Autodesk Inventor part; units mm, degrees
ref_plane "YZ Plane" through (0, 0, 0) normal (1, 0, 0) x (0, 1, 0)
ref_plane "XZ Plane" through (0, 0, 0) normal (0, 1, 0) x (-1, 0, 0)
ref_plane "XY Plane" through (0, 0, 0) normal (0, 0, 1) x (1, 0, 0)
sketch "Sketch1" plane through (0, 0, 0) normal (0, 0, 1) x (1, 0, 0)
  point P0 (0, 0)
sketch "Sketch2" plane through (0, 0, 0) normal (0, 0, 1) x (1, 0, 0)
  line L0 (-52.4998, -67.5002) -> (52.4998, -67.5002)
  line L1 (52.4998, -67.5002) -> (52.4998, 67.5002)
  line L2 (52.4998, 67.5002) -> (-52.4998, 67.5002)
  line L3 (-52.4998, 67.5002) -> (-52.4998, -67.5002)
  circle A0 centre (48, 60) radius 1.5002
  circle A1 centre (-48, 60) radius 1.5002
  circle A2 centre (-48, -60) radius 1.5002
  circle A3 centre (48, -60) radius 1.5002
  circle A4 centre (22, 60) radius 1.4999
  circle A5 centre (-22, 60) radius 1.4999
  circle A6 centre (22, -60) radius 1.4999
  circle A7 centre (-22, -60) radius 1.4999
  line L4 (0, -44.9999) -> (0, 44.9999)
  line L5 (30, -44.9999) -> (30, 44.9999)
  line L6 (30, 44.9999) -> (52.4998, 54.3179)
  line L7 (30, -44.9999) -> (52.4998, -54.3208)
  line L8 (-30, -44.9999) -> (-30, 44.9999)
  line L9 (-30, 44.9999) -> (-52.4998, 54.3179)
  line L10 (-30, -44.9999) -> (-52.4998, -54.3208)
extrude "Extrusion3" add sketch "Sketch2" along normal blind 3
fillet "Fillet4" radius 4 4 edges at (-52.4998, 67.5002, 1.5) (52.4998, 67.5002, 1.5) (52.4998, -67.5002, 1.5) (-52.4998, -67.5002, 1.5)
extrude "Extrusion4" cut sketch "Sketch2" along normal blind 10 contours L3 L9 L8 L10 | L7 L5 L6 L1
fillet "Fillet5" radius 4 8 edges at (52.4998, 54.3179, 1.5) (30, 44.9999, 1.5) (-30, 44.9999, 1.5) (-52.4998, 54.3179, 1.5) (-30, -44.9999, 1.5) (-52.4998, -54.3208, 1.5) (30, -44.9999, 1.5) (52.4998, -54.3208, 1.5)
properties part number "Controller - Power Board v2"
Part model, mm, in its own coordinate system. A direction names the side the tool comes from. Coordinates: 2 decimals unless noted, no trailing zeros. Write each loop counter-clockwise with the first axis right and the second up, starting at its lowest first coordinate (ties: lowest second). Pieces come first, ordered by that corner, then holes. Notation, with made-up numbers: M -19,74 L 37,74 A24 cw 37,102 Z; hole C -12,-15.75 d11. An arc over 180 degrees is marked long. Return JSON: item names as keys, results as strings.
1. Flat gauge pins, fed straight in: pin 1 Ø2.5 at (x, y) = (-48, 60) entering from -Z; pin 2 Ø1 at (y, z) = (-18, 2.5) entering from -X. Where does each tip first touch, or does it go through?
Determined:
{"pin 1": "through", "pin 2": "x = -30"}
2. Probe L1, parallel to Y at x = 22, z = 0.95; L2, parallel to Y at x = 48, z = 1.55; L3, parallel to X at y = 59, z = 0.3. List the from-to ranges inside material, lowest first.
Determined:
{"L1": "-67.5 to -61.5, -58.5 to 58.5, 61.5 to 67.5", "L2": "-67.5 to -61.5, -58.5 to -52.46, 52.45 to 58.5, 61.5 to 67.5", "L3": "-52.5 to -49.12, -46.88 to -23.12, -20.88 to 20.88, 23.12 to 46.88, 49.12 to 52.5"}
3. 3-axis set-ups, long thin cutter, end or side, ignore diameter. For faces 1 (the face through (-51.297, 66.36, 1.521)), 2 (the face through (-30, -1, 1)), 3 (the face through (30, -1, 1)): which of +Z, -Z, +X, -X, +Y, -Y reach the whole face in a straight line?
Determined:
{"face 1": "+Z, -Z, -X, +Y", "face 2": "+Z, -Z, -X", "face 3": "+Z, -Z, +X"}
4. Saw through at B-B, the plane y = -60. Write the cut outline in (x, z).
Determined:
{"outline": "M -52.5,0 L -49.5,0 L -49.5,3 L -52.5,3 Z; M -46.5,0 L -23.5,0 L -23.5,3 L -46.5,3 Z; M -20.5,0 L 20.5,0 L 20.5,3 L -20.5,3 Z; M 23.5,0 L 46.5,0 L 46.5,3 L 23.5,3 Z; M 49.5,0 L 52.5,0 L 52.5,3 L 49.5,3 Z"}
5. Saw through at A-A, the plane x = -22. Write the cut outline in (y, z), then the cut area to 3 significant figures.
Determined:
{"outline": "M -67.5,0 L -61.5,0 L -61.5,3 L -67.5,3 Z; M -58.5,0 L 58.5,0 L 58.5,3 L -58.5,3 Z; M 61.5,0 L 67.5,0 L 67.5,3 L 61.5,3 Z", "area": "387 mm²"}
6. Saw through at D-D, the plane x = 34.5. Write the cut outline in (y, z), then the cut area to 3 significant figures.
Determined:
{"outline": "M -67.5,0 L -46.86,0 L -46.86,3 L -67.5,3 Z; M 46.86,0 L 67.5,0 L 67.5,3 L 46.86,3 Z", "area": "124 mm²"}
7. Saw through at C-C, the plane z = 1.65. Count the separate pieces of the cut face and the enclosed holes in it, then the cut area to 3 significant figures.
Determined:
{"separate pieces": "1", "enclosed holes": "8", "area": "9,640 mm²"}
8. Pull direction X, two halves, no side cores. Call faces 4 (the face through (51.359, 66.297, 1.521)), 5 (the face through (-1, 1, 3)), 6 (the face through (47.805, -61.487, 1.479)): pulls with the +X half, pulls with the -X half, needs draft (parallel to the pull), parting line crosses it, or undercut.
Determined:
{"face 4": "pulls with the +X half", "face 5": "needs draft", "face 6": "undercut"}
